from build123d import *

# Parameters (mm, degrees)
SKETCH2_R          = 1
CUT_EXTRUDE1_DEPTH = 5


with BuildPart() as part:
    # Sketch1 → Revolve2 (revolve)
    with BuildSketch(Plane.XY):
        with BuildLine():
            Line((0, 2), (3, 2))
            Line((3, 2), (3, 1))
            Line((3, 1), (2.557179677, 0.744337567))
            ThreePointArc((2.557179677, 0.744337567), (2.374166975, 0.561324865), (2.307179677, 0.311324865))
            Line((2.307179677, 0.311324865), (2.307179677, -0.311324865))
            ThreePointArc((2.307179677, -0.311324865), (2.374166975, -0.561324865), (2.557179677, -0.744337567))
            Line((2.557179677, -0.744337567), (3, -1))
            Line((3, -1), (3, -2))
            Line((3, -2), (0, -2))
            Line((0, -2), (0, 2))
        make_face()
    revolve(axis=Axis((0, -2, 0), (0, 1, 0)))

    # Sketch2 → Cut-Extrude1 (cut, through all)
    with BuildSketch(Plane(origin=(0, 2, 0), x_dir=(1, 0, 0), z_dir=(0, 1, 0))):
        Circle(SKETCH2_R)
    extrude(amount=-CUT_EXTRUDE1_DEPTH, mode=Mode.SUBTRACT)


solid = part.part
Check sheet for the modelled part. Datum: model origin and axes. Units: mm. Round coordinates to 2 decimals unless told otherwise and drop trailing zeros. Loops run counter-clockwise (first coordinate to the right, second up) from the corner with the lowest first, then second, coordinate; pieces in that order, holes last. Notation, with made-up numbers: (-4.75, -10.5) - (41.25, -10.5) arc R32 cw to (41.25, 23.5) - close; hole circle Ø6 at (58, 16.5). An arc over 180 degrees is marked (long way). Answer as CSV lines item,"result". Start each with the question number.
Item 1: Section check B-B (z = 0). Record the boundary of the cut face in (x, y).
Item 2: Section check A-A (x = 0). Record the boundary of the cut face in (y, z), and give its area (3 significant figures).
Item 3: Depth check by flat-ended pin: P1, Ø2, axis at y = 1, z = -2.5, coming from the -X side. Enter the tip coordinate at first touch or a pass-through.
Item 4: Release check for a two-part mould opening along Y. For faces 1 (the cylindrical face through (-3, 1.5, -0.1)), 2 (the cylindrical face through (2.2, 0, -0.7)), 3 (the flat face through (-1, -2, -1)) record: +Y half, -Y half, draft (parallel to the pull), parting line (faces both ways), or undercut.
Item 5: Section check D-D (y = -0.85). Record the boundary of the cut face in (x, z), and give its area (3 significant figures).
Item 6: Section check C-C (y = 0.1). Record the boundary of the cut face in (x, z).
Item 7: Scan lines: line 1 (X direction, y = 0, z = 0); line 2 (X direction, y = 0.95, z = -0.5). Record each from-to range of solid material in increasing order. Write a range as [from, to].
Report:
1,outline,"(-3, -2) - (-1, -2) - (-1, 2) - (-3, 2) - (-3, 1) - (-2.56, 0.74) arc R0.5 cw to (-2.31, 0.31) - (-2.31, -0.31) arc R0.5 cw to (-2.56, -0.74) - (-3, -1) - close; (1, -2) - (3, -2) - (3, -1) - (2.56, -0.74) arc R0.5 cw to (2.31, -0.31) - (2.31, 0.31) arc R0.5 cw to (2.56, 0.74) - (3, 1) - (3, 2) - (1, 2) - close"
2,outline,"(-2, -3) - (-1, -3) - (-0.74, -2.56) arc R0.5 cw to (-0.31, -2.31) - (0.31, -2.31) arc R0.5 cw to (0.74, -2.56) - (1, -3) - (2, -3) - (2, -1) - (-2, -1) - close; (-2, 1) - (2, 1) - (2, 3) - (1, 3) - (0.74, 2.56) arc R0.5 cw to (0.31, 2.31) - (-0.31, 2.31) arc R0.5 cw to (-0.74, 2.56) - (-1, 3) - (-2, 3) - close"
2,area,"13.8 mm2"
3,P1,"stops at x = -2.6"
4,face 1,"draft"
4,face 2,"undercut"
4,face 3,"-Y half"
5,outline,"circle Ø5.48 at (0, 0); hole circle Ø2 at (0, 0)"
5,area,"20.4 mm2"
6,outline,"circle Ø4.61 at (0, 0); hole circle Ø2 at (0, 0)"
7,line 1,"x = [-2.31, -1], [1, 2.31]"
7,line 2,"x = [-2.87, -0.87], [0.87, 2.87]"
